Autodesk Inventor part; units mm, degrees
ref_plane "YZ Plane" through (0, 0, 0) normal (1, 0, 0) x (0, 1, 0)
ref_plane "XZ Plane" through (0, 0, 0) normal (0, 1, 0) x (-1, 0, 0)
ref_plane "XY Plane" through (0, 0, 0) normal (0, 0, 1) x (1, 0, 0)
sketch "スケッチ1" plane through (0, 0, 0) normal (1, 0, 0) x (0, 1, 0)
  arc A0 (17.1756, 0.6715) -> (-15.9786, -6.3353) centre (0, 0) ccw
  arc A1 (-34.1332, -435.9093) -> (34.3512, -438.657) centre (0, -440) ccw
  arc A2 (9.3592, -73.0018) -> (8.8263, -68.897) centre (1, -72) ccw
  line L0 (8.8263, -68.897) -> (-15.9786, -6.3353)
  line L1 (34.3512, -438.657) -> (17.1756, 0.6715)
  line L2 (9.3592, -73.0018) -> (-34.1332, -435.9093)
  arc A3 (17.5943, 0.6879) -> (-16.3681, -6.4898) centre (0, 0) ccw
  line L3 (-16.3681, -6.4898) -> (8.4368, -69.0514)
  arc A4 (8.9432, -72.9519) -> (8.4368, -69.0514) centre (1, -72) ccw
  line L4 (8.9432, -72.9519) -> (-34.5492, -435.8595)
  arc A5 (-34.5492, -435.8595) -> (34.7699, -438.6407) centre (0, -440) ccw
  line L5 (34.7699, -438.6407) -> (17.5943, 0.6879)
  arc A6 (16.7949, 0.6566) -> (-15.6244, -6.1949) centre (0, 0) ccw
  line L6 (-15.6244, -6.1949) -> (9.1805, -68.7565)
  arc A7 (9.7375, -73.0471) -> (9.1805, -68.7565) centre (1, -72) ccw
  line L7 (9.7375, -73.0471) -> (-33.7549, -435.9547)
  arc A8 (-33.7549, -435.9547) -> (33.9705, -438.6719) centre (0, -440) ccw
  line L8 (33.9705, -438.6719) -> (16.7949, 0.6566)
  dimension "d0" = 34.3775
  dimension "d1" = 68.7549
  dimension "d2" = 440
  dimension "d24" = 0.419
  dimension "d25" = 8
  dimension "d26" = 72
  dimension "d27" = 0.8
  dimension "d32" = 1
extrude "押し出し1" add sketch "スケッチ1" along normal mid plane 10 contours L1 A1 L2 A2 L0 A0 | L5 A5 L4 A4 L3 A3
properties part number "belt_2" material "ゴム"
For this review, take the finished solid that the model builds, in its own axes (mm). A direction names the side the tool comes from. Coordinates: 2 decimals unless noted, no trailing zeros. Order: outer loops, then holes, each group sorted by start corner. A loop starts at its lowest first (then second) coordinate and runs counter-clockwise, first axis right, second up. Notation, with made-up numbers: (30, 36) - (73, 36) arc R13 ccw to (73, 46) - close; hole circle Ø6 at (16.25, 16.5). An arc over 180 degrees is marked (long way). Use one line per item in the form item = value.
Q1. For probe 1 along Y at (x, z) = (-4.5, -417.5); probe 2 along Y at (x, z) = (0, -389), list the stretches that pass through material, from the lowest coordinate up. Write a range as from..to.
Checked values:
probe_1 = -32.35..-31.54, 33.14..33.94
probe_2 = -28.93..-28.13, 32.03..32.83
Q2. Draft analysis for pull direction Y (two halves, no side actions). For faces 4 (the flat face through (0.07, -12.5, -251.87)), 5 (the flat face through (0.07, 25.503, -222.083)), 6 (the cylindrical face through (0.07, -2.198, -474.727)), state which applies: +Y half, -Y half, draft (parallel to the pull), parting line (faces both ways), or undercut.
Checked values:
face_4 = -Y half
face_5 = undercut
face_6 = parting line
Q3. Consider section A-A (x = -2.5). Give the boundary of the cut face in (y, z), then the cut area to 3 significant figures.
Checked values:
outline = (-34.55, -435.86) arc R34.8 ccw (long way) to (34.77, -438.64) - (17.59, 0.69) arc R17.61 ccw (long way) to (-16.37, -6.49) - (8.44, -69.05) arc R8 cw to (8.94, -72.95) - close; hole (-33.75, -435.95) arc R34 ccw (long way) to (33.97, -438.67) - (16.79, 0.66) arc R16.81 ccw (long way) to (-15.62, -6.19) - (9.18, -68.76) arc R8.8 cw to (9.74, -73.05) - close
area = 840 mm2
Q4. Consider section D-D (z = -153.5). Give the boundary of the cut face in (x, y), then the cut area to 3 significant figures.
Checked values:
outline = (-5, -0.71) - (5, -0.71) - (5, 0.1) - (-5, 0.1) - close; (-5, 22.82) - (5, 22.82) - (5, 23.62) - (-5, 23.62) - close
area = 16.1 mm2
Q5. For faces 1 (the flat face through (0.07, -4.14, -37.33)), 2 (the flat face through (0.07, -3.396, -37.038)), 3 (the flat face through (5, 25.6, -209.2)), list the 3-axis set-ups (+Z, -Z, +X, -X, +Y, -Y) from which the entire face can be reached by the end or side of a thin tool; tool diameter is ignored.
Checked values:
face_1 = +X, -X, -Y
face_2 = +X, -X
face_3 = +Z, -Z, +X, +Y, -Y
Q6. Consider section B-B (y = -8.5). Give the boundary of the cut face in (x, z), then the cut area to 3 significant figures.
Checked values:
outline = (-5, -473.74) - (5, -473.74) - (5, -472.92) - (-5, -472.92) - close; (-5, -225.22) - (5, -225.22) - (5, -218.5) - (-5, -218.5) - close; (-5, -26.33) - (5, -26.33) - (5, -24.16) - (-5, -24.16) - close; (-5, 14.5) - (5, 14.5) - (5, 15.42) - (-5, 15.42) - close
area = 106 mm2
Q7. For P1, Ø4, axis at x = -3.5, y = 3, coming from the -Z side; P2, Ø1.5, axis at x = 2.5, y = -5.5, coming from the -Z side; P3, Ø5, axis at x = 2, z = -108.5, coming from the -Y side, all flat-tipped, find the tip position at first contact; note any pin that passes through.
Checked values:
P1 = -474.78
P2 = -474.47
P3 = 4.38
Q8. Consider section C-C (y = 26). Give the boundary of the cut face in (x, z).
Checked values:
outline = (-5, -463.13) - (5, -463.13) - (5, -461.9) - (-5, -461.9) - close; (-5, -234.8) - (5, -234.8) - (5, -214.32) - (-5, -214.32) - close
